Read the model definition and answer for the solid it produces. Units are mm, in the model's axes. A direction names the side the tool comes from. Coordinates: 2 decimals unless noted, no trailing zeros. Order: outer loops, then holes, each group sorted by start corner. A loop starts at its lowest first (then second) coordinate and runs counter-clockwise, first axis right, second up. Notation, with made-up numbers: M 62,-23.75 L 84,-23.75 A6 ccw 84,-13.75 Z; hole C -1,36 d9. An arc over 180 degrees is marked long. One line per question, with ' | ' between items. Start each with the question number.
1) Find section D-D, the plane x = -2.25. Write down the section's boundary in (y, z), plus the area to 3 significant figures.
2) Find section B-B, the plane z = 1.7. Count the separate pieces of the cut face and the enclosed holes in it, plus the area to 3 significant figures.
3) Consider probe 1 along Y at (x, z) = (-0.5, 0.3); probe 2 along X at (y, z) = (7.75, 0.15); probe 3 along Z at (x, y) = (2.5, -4.5). Determine where each line is inside the solid, lowest interval first.
4) Find section C-C, the plane y = 1. Write down the section's boundary in (x, z), plus the area to 3 significant figures.
5) A tool of negligible diameter and unlimited length cuts with its end or side. For faces 1 (the face through (-7, -7.75, 1)), 2 (the face through (0, 0, 2)), 3 (the face through (-2.605, 0, -2)), 4 (the face through (1, 2.141, -2)), 5 (the face through (1, -2.138, -2)), from which of +Z, -Z, +X, -X, +Y, -Y can it reach the whole face along a straight path? Write none if from no direction.
6) Find section A-A, the plane y = 7. Write down the section's boundary in (x, z), plus the area to 3 significant figures.
7) Given P1, Ø1.6, axis at x = 2.5, z = -2, coming from the -Y side; P2, Ø0.6, axis at y = 1, z = 1, coming from the -X side; P3, Ø1.6, axis at x = -6, z = 1, coming from the +Y side, each flat-ended and moving along its own axis, determine where each tip first touches the part or whether it passes through.
8) The mould has two halves that part along Y. Classify faces 6 (the face through (0.958, 8.867, 0.986)), 7 (the face through (0, 11.75, 1)), 8 (the face through (5, 0, 1)): +Y half, -Y half, draft (parallel to the pull), parting line (faces both ways), or undercut.
Autodesk Inventor part; units mm, degrees
ref_plane "РабПлоскость1" through (-4.9754, -3.7735, -3.25) normal (0, 0, 1) x (1, 0, 0)
ref_plane "YZ Plane" through (0, 0, 0) normal (1, 0, 0) x (0, 1, 0)
ref_plane "XZ Plane" through (0, 0, 0) normal (0, 1, 0) x (-1, 0, 0)
sketch "Эскиз1" plane through (0, 0, 0) normal (0, 0, 1) x (1, 0, 0)
  circle A0 centre (0.3813, 7.7585) radius 1.25
  line L0 (-4.9754, 3.7665) -> (-4.9754, 11.75)
  line L1 (5, 3.7665) -> (-4.9754, 3.7665)
  line L2 (5, 11.75) -> (5, 3.7665)
  line L3 (-4.9754, 11.75) -> (5, 11.75)
  arc A1 (1.6313, -7.75) -> (-0.8686, -7.75) centre (0.3813, -7.762) ccw
  line L4 (-0.8686, -7.75) -> (1.6313, -7.75)
  line L5 (5, -11.75) -> (-8, -11.75)
  line L6 (5, -3.7735) -> (5, -11.75)
  line L7 (-5, -3.7735) -> (5, -3.7735)
  line L8 (-5, -7.75) -> (-5, -3.7735)
  line L9 (-8, -7.75) -> (-5, -7.75)
  line L10 (-8, -11.75) -> (-8, -7.75)
  line L11 (3.0114, -0.7535) -> (3.0052, -0.7535)
  line L12 (3.0114, -0.7535) -> (3.0114, -0.7535)
  arc A2 (3.5595, -1.3518) -> (3.0114, -0.7535) centre (3.0062, -1.3085) ccw
  arc A3 (3.5595, -1.3518) -> (3.709, -1.5135) centre (3.709, -1.3635) ccw
  line L13 (4.3002, -1.5135) -> (3.709, -1.5135)
  arc A4 (4.3002, -1.5135) -> (4.4502, -1.3635) centre (4.3002, -1.3635) ccw
  line L14 (4.4502, -1.2761) -> (4.4502, -1.3635)
  line L15 (4.4521, -1.2761) -> (4.4502, -1.2761)
  arc A5 (5, -0.7535) -> (4.4521, -1.2761) centre (5.0062, -1.3085) ccw
  line L16 (5, 0.7465) -> (5, -0.7535)
  arc A6 (4.4521, 1.2691) -> (5, 0.7465) centre (5.0062, 1.3015) ccw
  line L17 (4.4502, 1.2691) -> (4.4521, 1.2691)
  line L18 (4.4502, 1.3565) -> (4.4502, 1.2691)
  arc A7 (4.4502, 1.3565) -> (4.3002, 1.5065) centre (4.3002, 1.3565) ccw
  line L19 (3.709, 1.5065) -> (4.3002, 1.5065)
  arc A8 (3.709, 1.5065) -> (3.5595, 1.3448) centre (3.709, 1.3565) ccw
  arc A9 (3.0114, 0.7465) -> (3.5595, 1.3448) centre (3.0062, 1.3015) ccw
  line L20 (3.0114, 0.7465) -> (3.0114, 0.7465)
  line L21 (3.0052, 0.7465) -> (3.0114, 0.7465)
  line L22 (3.0052, 0.7465) -> (3.0052, 0.7465)
  arc A10 (2.4583, 1.2691) -> (3.0052, 0.7465) centre (3.0123, 1.3015) ccw
  line L23 (2.4564, 1.2691) -> (2.4583, 1.2691)
  line L24 (2.4564, 1.3565) -> (2.4564, 1.2691)
  arc A11 (2.4564, 1.3565) -> (2.3064, 1.5065) centre (2.3064, 1.3565) ccw
  line L25 (1.7152, 1.5065) -> (2.3064, 1.5065)
  arc A12 (1.7152, 1.5065) -> (1.5656, 1.3448) centre (1.7152, 1.3565) ccw
  arc A13 (1.0175, 0.7465) -> (1.5656, 1.3448) centre (1.0123, 1.3015) ccw
  line L26 (1.0175, 0.7465) -> (1.0175, 0.7465)
  line L27 (1.0114, 0.7465) -> (1.0175, 0.7465)
  line L28 (1.0114, 0.7465) -> (1.0114, 0.7465)
  arc A14 (0.4644, 1.2691) -> (1.0114, 0.7465) centre (1.0185, 1.3015) ccw
  line L29 (0.4625, 1.2691) -> (0.4644, 1.2691)
  line L30 (0.4625, 1.3565) -> (0.4625, 1.2691)
  arc A15 (0.4625, 1.3565) -> (0.3125, 1.5065) centre (0.3125, 1.3565) ccw
  line L31 (-0.2787, 1.5065) -> (0.3125, 1.5065)
  arc A16 (-0.2787, 1.5065) -> (-0.4282, 1.3448) centre (-0.2787, 1.3565) ccw
  arc A17 (-0.9763, 0.7465) -> (-0.4282, 1.3448) centre (-0.9815, 1.3015) ccw
  line L32 (-0.9763, 0.7465) -> (-0.9763, 0.7465)
  line L33 (-0.9825, 0.7465) -> (-0.9763, 0.7465)
  line L34 (-0.9825, 0.7465) -> (-0.9825, 0.7465)
  arc A18 (-1.5294, 1.2691) -> (-0.9825, 0.7465) centre (-0.9754, 1.3015) ccw
  line L35 (-1.5313, 1.2691) -> (-1.5294, 1.2691)
  line L36 (-1.5313, 1.3565) -> (-1.5313, 1.2691)
  arc A19 (-1.5313, 1.3565) -> (-1.6813, 1.5065) centre (-1.6813, 1.3565) ccw
  line L37 (-2.2725, 1.5065) -> (-1.6813, 1.5065)
  arc A20 (-2.2725, 1.5065) -> (-2.4221, 1.3448) centre (-2.2725, 1.3565) ccw
  arc A21 (-2.9754, 0.7465) -> (-2.4221, 1.3448) centre (-2.9754, 1.3015) ccw
  line L38 (-2.9754, 0.7465) -> (-2.9754, 2.2665)
  line L39 (5, 2.2665) -> (-2.9754, 2.2665)
  line L40 (5, 3.7665) -> (5, 2.2665)
  line L41 (-4.9754, 3.7665) -> (5, 3.7665)
  line L42 (-4.9754, -3.7735) -> (-4.9754, 3.7665)
  line L43 (5, -3.7735) -> (-4.9754, -3.7735)
  line L44 (5, -2.2735) -> (5, -3.7735)
  line L45 (-2.9754, -2.2735) -> (5, -2.2735)
  line L46 (-2.9754, -2.2735) -> (-2.9754, -0.7535)
  arc A22 (-2.4221, -1.3518) -> (-2.9754, -0.7535) centre (-2.9754, -1.3085) ccw
  arc A23 (-2.4221, -1.3518) -> (-2.2725, -1.5135) centre (-2.2725, -1.3635) ccw
  line L47 (-1.6813, -1.5135) -> (-2.2725, -1.5135)
  arc A24 (-1.6813, -1.5135) -> (-1.5313, -1.3635) centre (-1.6813, -1.3635) ccw
  line L48 (-1.5313, -1.2761) -> (-1.5313, -1.3635)
  line L49 (-1.5294, -1.2761) -> (-1.5313, -1.2761)
  arc A25 (-0.9825, -0.7535) -> (-1.5294, -1.2761) centre (-0.9754, -1.3085) ccw
  line L50 (-0.9825, -0.7535) -> (-0.9825, -0.7535)
  line L51 (-0.9763, -0.7535) -> (-0.9825, -0.7535)
  line L52 (-0.9763, -0.7535) -> (-0.9763, -0.7535)
  arc A26 (-0.4282, -1.3518) -> (-0.9763, -0.7535) centre (-0.9815, -1.3085) ccw
  arc A27 (-0.4282, -1.3518) -> (-0.2787, -1.5135) centre (-0.2787, -1.3635) ccw
  line L53 (0.3125, -1.5135) -> (-0.2787, -1.5135)
  arc A28 (0.3125, -1.5135) -> (0.4625, -1.3635) centre (0.3125, -1.3635) ccw
  line L54 (0.4625, -1.2761) -> (0.4625, -1.3635)
  line L55 (0.4644, -1.2761) -> (0.4625, -1.2761)
  arc A29 (1.0114, -0.7535) -> (0.4644, -1.2761) centre (1.0185, -1.3085) ccw
  line L56 (1.0114, -0.7535) -> (1.0114, -0.7535)
  line L57 (1.0175, -0.7535) -> (1.0114, -0.7535)
  line L58 (1.0175, -0.7535) -> (1.0175, -0.7535)
  arc A30 (1.5656, -1.3518) -> (1.0175, -0.7535) centre (1.0123, -1.3085) ccw
  arc A31 (1.5656, -1.3518) -> (1.7152, -1.5135) centre (1.7152, -1.3635) ccw
  line L59 (2.3064, -1.5135) -> (1.7152, -1.5135)
  arc A32 (2.3064, -1.5135) -> (2.4564, -1.3635) centre (2.3064, -1.3635) ccw
  line L60 (2.4564, -1.2761) -> (2.4564, -1.3635)
  line L61 (2.4583, -1.2761) -> (2.4564, -1.2761)
  arc A33 (3.0052, -0.7535) -> (2.4583, -1.2761) centre (3.0123, -1.3085) ccw
  line L62 (3.0052, -0.7535) -> (3.0052, -0.7535)
  circle A34 centre (0.3813, -7.762) radius 1.25
  line L63 (5, 2.2665) -> (5, -2.2735)
  point P0 (0, 0)
  point P1 (5, -0.7535)
  point P2 (-0.8686, -7.75)
extrude "Выдавливание1" add sketch "Эскиз1" along normal blind 2
sketch "Эскиз2" plane through (0, 0, 0) normal (0, 0, -1) x (-1, 0, 0)
  line L0 (-5, 2.2665) -> (-5, 0.7465)
  line L1 (-3.0114, -0.7535) -> (-3.0052, -0.7535)
  line L2 (-3.0114, -0.7535) -> (-3.0114, -0.7535)
  arc A0 (-3.0114, -0.7535) -> (-3.5595, -1.3518) centre (-3.0062, -1.3085) ccw
  arc A1 (-3.709, -1.5135) -> (-3.5595, -1.3518) centre (-3.709, -1.3635) ccw
  line L3 (-4.3002, -1.5135) -> (-3.709, -1.5135)
  arc A2 (-4.4502, -1.3635) -> (-4.3002, -1.5135) centre (-4.3002, -1.3635) ccw
  line L4 (-4.4502, -1.2761) -> (-4.4502, -1.3635)
  line L5 (-4.4521, -1.2761) -> (-4.4502, -1.2761)
  arc A3 (-4.4521, -1.2761) -> (-5, -0.7535) centre (-5.0062, -1.3085) ccw
  line L6 (-5, 0.7465) -> (-5, -0.7535)
  arc A4 (-5, 0.7465) -> (-4.4521, 1.2691) centre (-5.0062, 1.3015) ccw
  line L7 (-4.4502, 1.2691) -> (-4.4521, 1.2691)
  line L8 (-4.4502, 1.3565) -> (-4.4502, 1.2691)
  arc A5 (-4.3002, 1.5065) -> (-4.4502, 1.3565) centre (-4.3002, 1.3565) ccw
  line L9 (-3.709, 1.5065) -> (-4.3002, 1.5065)
  arc A6 (-3.5595, 1.3448) -> (-3.709, 1.5065) centre (-3.709, 1.3565) ccw
  arc A7 (-3.5595, 1.3448) -> (-3.0114, 0.7465) centre (-3.0062, 1.3015) ccw
  line L10 (-3.0114, 0.7465) -> (-3.0114, 0.7465)
  line L11 (-3.0052, 0.7465) -> (-3.0114, 0.7465)
  line L12 (-3.0052, 0.7465) -> (-3.0052, 0.7465)
  arc A8 (-3.0052, 0.7465) -> (-2.4583, 1.2691) centre (-3.0123, 1.3015) ccw
  line L13 (-2.4564, 1.2691) -> (-2.4583, 1.2691)
  line L14 (-2.4564, 1.3565) -> (-2.4564, 1.2691)
  arc A9 (-2.3064, 1.5065) -> (-2.4564, 1.3565) centre (-2.3064, 1.3565) ccw
  line L15 (-1.7152, 1.5065) -> (-2.3064, 1.5065)
  arc A10 (-1.5656, 1.3448) -> (-1.7152, 1.5065) centre (-1.7152, 1.3565) ccw
  arc A11 (-1.5656, 1.3448) -> (-1.0175, 0.7465) centre (-1.0123, 1.3015) ccw
  line L16 (-1.0175, 0.7465) -> (-1.0175, 0.7465)
  line L17 (-1.0114, 0.7465) -> (-1.0175, 0.7465)
  line L18 (-1.0114, 0.7465) -> (-1.0114, 0.7465)
  arc A12 (-1.0114, 0.7465) -> (-0.4644, 1.2691) centre (-1.0185, 1.3015) ccw
  line L19 (-0.4625, 1.2691) -> (-0.4644, 1.2691)
  line L20 (-0.4625, 1.3565) -> (-0.4625, 1.2691)
  arc A13 (-0.3125, 1.5065) -> (-0.4625, 1.3565) centre (-0.3125, 1.3565) ccw
  line L21 (0.2787, 1.5065) -> (-0.3125, 1.5065)
  arc A14 (0.4282, 1.3448) -> (0.2787, 1.5065) centre (0.2787, 1.3565) ccw
  arc A15 (0.4282, 1.3448) -> (0.9763, 0.7465) centre (0.9815, 1.3015) ccw
  line L22 (0.9763, 0.7465) -> (0.9763, 0.7465)
  line L23 (0.9825, 0.7465) -> (0.9763, 0.7465)
  line L24 (0.9825, 0.7465) -> (0.9825, 0.7465)
  arc A16 (0.9825, 0.7465) -> (1.5294, 1.2691) centre (0.9754, 1.3015) ccw
  line L25 (1.5313, 1.2691) -> (1.5294, 1.2691)
  line L26 (1.5313, 1.3565) -> (1.5313, 1.2691)
  arc A17 (1.6813, 1.5065) -> (1.5313, 1.3565) centre (1.6813, 1.3565) ccw
  line L27 (2.2725, 1.5065) -> (1.6813, 1.5065)
  arc A18 (2.4221, 1.3448) -> (2.2725, 1.5065) centre (2.2725, 1.3565) ccw
  arc A19 (2.4221, 1.3448) -> (2.9754, 0.7465) centre (2.9754, 1.3015) ccw
  line L28 (2.9754, 0.7465) -> (2.9754, 2.2665)
  line L29 (-5, 2.2665) -> (2.9754, 2.2665)
  line L30 (-5, 3.7665) -> (-5, 2.2665)
  line L31 (4.9754, 3.7665) -> (-5, 3.7665)
  line L32 (4.9754, -3.7735) -> (4.9754, 3.7665)
  line L33 (-5, -3.7735) -> (4.9754, -3.7735)
  line L34 (-5, -2.2735) -> (-5, -3.7735)
  line L35 (2.9754, -2.2735) -> (-5, -2.2735)
  line L36 (2.9754, -2.2735) -> (2.9754, -0.7535)
  arc A20 (2.9754, -0.7535) -> (2.4221, -1.3518) centre (2.9754, -1.3085) ccw
  arc A21 (2.2725, -1.5135) -> (2.4221, -1.3518) centre (2.2725, -1.3635) ccw
  line L37 (1.6813, -1.5135) -> (2.2725, -1.5135)
  arc A22 (1.5313, -1.3635) -> (1.6813, -1.5135) centre (1.6813, -1.3635) ccw
  line L38 (1.5313, -1.2761) -> (1.5313, -1.3635)
  line L39 (1.5294, -1.2761) -> (1.5313, -1.2761)
  arc A23 (1.5294, -1.2761) -> (0.9825, -0.7535) centre (0.9754, -1.3085) ccw
  line L40 (0.9825, -0.7535) -> (0.9825, -0.7535)
  line L41 (0.9763, -0.7535) -> (0.9825, -0.7535)
  line L42 (0.9763, -0.7535) -> (0.9763, -0.7535)
  arc A24 (0.9763, -0.7535) -> (0.4282, -1.3518) centre (0.9815, -1.3085) ccw
  arc A25 (0.2787, -1.5135) -> (0.4282, -1.3518) centre (0.2787, -1.3635) ccw
  line L43 (-0.3125, -1.5135) -> (0.2787, -1.5135)
  arc A26 (-0.4625, -1.3635) -> (-0.3125, -1.5135) centre (-0.3125, -1.3635) ccw
  line L44 (-0.4625, -1.2761) -> (-0.4625, -1.3635)
  line L45 (-0.4644, -1.2761) -> (-0.4625, -1.2761)
  arc A27 (-0.4644, -1.2761) -> (-1.0114, -0.7535) centre (-1.0185, -1.3085) ccw
  line L46 (-1.0114, -0.7535) -> (-1.0114, -0.7535)
  line L47 (-1.0175, -0.7535) -> (-1.0114, -0.7535)
  line L48 (-1.0175, -0.7535) -> (-1.0175, -0.7535)
  arc A28 (-1.0175, -0.7535) -> (-1.5656, -1.3518) centre (-1.0123, -1.3085) ccw
  arc A29 (-1.7152, -1.5135) -> (-1.5656, -1.3518) centre (-1.7152, -1.3635) ccw
  line L49 (-2.3064, -1.5135) -> (-1.7152, -1.5135)
  arc A30 (-2.4564, -1.3635) -> (-2.3064, -1.5135) centre (-2.3064, -1.3635) ccw
  line L50 (-2.4564, -1.2761) -> (-2.4564, -1.3635)
  line L51 (-2.4583, -1.2761) -> (-2.4564, -1.2761)
  arc A31 (-2.4583, -1.2761) -> (-3.0052, -0.7535) centre (-3.0123, -1.3085) ccw
  line L52 (-3.0052, -0.7535) -> (-3.0052, -0.7535)
  line L53 (-5, -11.75) -> (-5, 11.75)
  line L54 (-5, -2.1382) -> (-5, 2.1409)
  line L55 (-5, -2.1382) -> (2.6046, -2.1382)
  line L56 (2.6046, -2.1382) -> (2.6046, 2.1409)
  line L57 (-5, 2.1409) -> (2.6046, 2.1409)
  line L58 (-5, -11.75) -> (-5, 11.75)
  point P0 (0, 0)
ref_plane "РабПлоскость1" through (-4.9754, -3.7735, -3.25) normal (0, 0, 1) x (1, 0, 0)
extrude "Выдавливание2" add sketch "Эскиз2" along normal up to surface (3.25 mm away) contours L57 L56 A19 A18 L27 A17 L26 A16 L23 A15 A14 L21 A13 L20 A12 L17 A11 A10 L15 A9 L14 A8 L11 A7 A6 L9 A5 L8 A4 L0 | A4 L8 A5 L9 A6 A7 L11 A8 L14 A9 L15 A10 A11 L17 A12 L20 A13 L21 A14 A15 L23 A16 L26 A17 L27 A18 A19 L56 A20 A21 L37 A22 L38 A23 L41 A24 A25 L43 A26 L44 A27 L47 A28 A29 L49 A30 L50 A31 L1 A0 A1 L3 A2 L4 A3 L6 | A3 L4 A2 L3 A1 A0 L1 A31 L50 A30 L49 A29 A28 L47 A27 L44 A26 L43 A25 A24 L41 A23 L38 A22 L37 A21 A20 L56 L55 L53
properties part number "крышка"
Report:
1) outline: M -11.75,0 L -2.14,0 L -2.14,-3.25 L 2.14,-3.25 L 2.14,0 L 11.75,0 L 11.75,2 L -11.75,2 Z | area: 60.9 mm^2
2) separate pieces: 1 | enclosed holes: 2 | area: 237 mm^2
3) probe 1: y = -11.75 to -8.65, -6.88 to 6.87, 8.64 to 11.75 | probe 2: x = -4.98 to -0.87, 1.63 to 5 | probe 3: z = 0 to 2
4) outline: M -4.98,0 L -2.6,0 L -2.6,-3.25 L 5,-3.25 L 5,2 L -4.98,2 Z | area: 44.7 mm^2
5) face 1: +Z, -Z, -X, +Y | face 2: +Z, +X, -X, +Y, -Y | face 3: -Z, -X, +Y, -Y | face 4: -Z, +X, -X, +Y | face 5: -Z, +X, -X, -Y
6) outline: M -4.98,0 L -0.61,0 L -0.61,2 L -4.98,2 Z; M 1.37,0 L 5,0 L 5,2 L 1.37,2 Z | area: 16.0 mm^2
7) P1: stops at y = -2.14 | P2: stops at x = -4.98 | P3: stops at y = -7.75
8) face 6: undercut | face 7: +Y half | face 8: draft
